from build123d import *

# Parameters (mm, degrees)
F0_W     = 90
F0_H     = 90
F0_R     = 2.6
F0_R_2   = 2.5
F0_R_3   = 7.5
F1_DEPTH = 7
F2_DEPTH = 10


# Not quite as in the source:
# - a feature names something its author has since deleted; it is built from what else it names


with BuildPart() as f1:
    # F0 (on Top) → F1 (new body)
    with BuildSketch(Plane.XY):
        Rectangle(F0_W, F0_H)
        with Locations((-28.2842712475, -28.2842712475)):
            Circle(F0_R, mode=Mode.SUBTRACT)
        with Locations((-29.9999999986, -0.0002877)):
            Circle(F0_R_2, mode=Mode.SUBTRACT)
        with Locations((28.2842712475, -28.2842712475)):
            Circle(F0_R, mode=Mode.SUBTRACT)
        with Locations((-28.2842712475, 28.2842712475)):
            Circle(F0_R, mode=Mode.SUBTRACT)
        Circle(F0_R_3, mode=Mode.SUBTRACT)
        with Locations((29.9999999986, 0.0002877)):
            Circle(F0_R_2, mode=Mode.SUBTRACT)
        with Locations((28.2842712475, 28.2842712475)):
            Circle(F0_R, mode=Mode.SUBTRACT)
        with Locations((-29.9999999986, -0.0002877)):
            Circle(F0_R_2)
        with Locations((29.9999999986, 0.0002877)):
            Circle(F0_R_2)
    extrude(amount=F1_DEPTH)

    # F0 (on Top) → F2 (join)
    with BuildSketch(Plane.XY):
        with Locations((29.9999999986, 0.0002877)):
            Circle(F0_R_2)
        with Locations((-29.9999999986, -0.0002877)):
            Circle(F0_R_2)
    extrude(amount=-F2_DEPTH)


solid = f1.part
Can you work these out from the model? Positions are in its coordinate system, mm. A direction names the side the tool comes from. Coordinates: 2 decimals unless noted, no trailing zeros. Order: outer loops, then holes, each group sorted by start corner. A loop starts at its lowest first (then second) coordinate and runs counter-clockwise, first axis right, second up. Notation, with made-up numbers: M -9.5,-12 L -5.5,-12 A31 cw -5.5,14 Z; hole C -0.5,-18 d8. An arc over 180 degrees is marked long. Answer as CSV lines item,"result".
(1) If we mould it in two halves opening along X, with no side actions, what happens to faces 3 (the flat face through (-1, 11, 7)), 4 (the cylindrical face through (27.5, 0.1, -4.9)), 5 (the flat face through (-45, -1, 3))? For each: released by +X, released by -X, zero draft, split by the parting line, or undercut.
Geometry check:
face 3,"zero draft"
face 4,"undercut"
face 5,"released by -X"
(2) Suppose I cut it at B-B on z = 5. Please give me the cut outline in (x, y), plus the area to 3 significant figures.
Geometry check:
outline,"M -45,-45 L 45,-45 L 45,45 L -45,45 Z; hole C -28.28,-28.28 d5.2; hole C -28.28,28.28 d5.2; hole C 0,0 d15; hole C 28.28,-28.28 d5.2; hole C 28.28,28.28 d5.2"
area,"7,840 mm^2"
(3) Suppose I cut it at A-A on x = 0. Please give me the cut outline in (y, z).
Geometry check:
outline,"M -45,0 L -7.5,0 L -7.5,7 L -45,7 Z; M 7.5,0 L 45,0 L 45,7 L 7.5,7 Z"
(4) On a 3-axis mill with a long thin cutter (end or side, diameter ignored), from which of +Z, -Z, +X, -X, +Y, -Y can I reach the whole of each face in a straight line? I mean faces 1 (the cylindrical face through (-26.89, 30.48, 3.45)), 2 (the cylindrical face through (-27.615, 0.751, -4.93)). Say none if no direction works.
Geometry check:
face 1,"+Z, -Z"
face 2,"-Z"
(5) Please list where these lines run through material, in increasing order: L1, parallel to Y at x = 0, z = 5.25; L2, parallel to X at y = 0, z = -5; L3, parallel to Z at x = -7, y = -31.
Geometry check:
L1,"-45 to -7.5, 7.5 to 45"
L2,"-32.5 to -27.5, 27.5 to 32.5"
L3,"0 to 7"
(6) I'm going to push a flat-ended pin straight in: pin 1 (8.5 mm diameter, centred on x = 28.28, y = 28.28, fed in from -Z). Where does the tip first touch, or does it pass through?
Geometry check:
pin 1,"z = 0"
(7) Suppose I cut it at C-C on y = 37. Please give me the cut outline in (x, z).
Geometry check:
outline,"M -45,0 L 45,0 L 45,7 L -45,7 Z"
